from build123d import *

# Parameters (mm, degrees)
BOSS_EXTRUDE1_DEPTH = 9.8
LPATTERN1_COUNT     = 20
LPATTERN1_PITCH     = 11


with BuildPart() as part:
    # Sketch1 → Boss-Extrude1 (new body)
    with BuildSketch(Plane(origin=(0, 0, 0), x_dir=(0, 0, -1), z_dir=(1, 0, 0))):
        Polygon((0, 0), (4.8, 0), (11, 0), (11, 2.8), (4.8, 2.8), (4.8, 5.8), (0, 5.8), align=None)
    boss_extrude1 = extrude(amount=BOSS_EXTRUDE1_DEPTH)

    # LPattern1: Boss-Extrude1 ×20
    with Locations(*[(0, 0, -i * LPATTERN1_PITCH) for i in range(1, LPATTERN1_COUNT)]):
        add(boss_extrude1)


solid = part.part
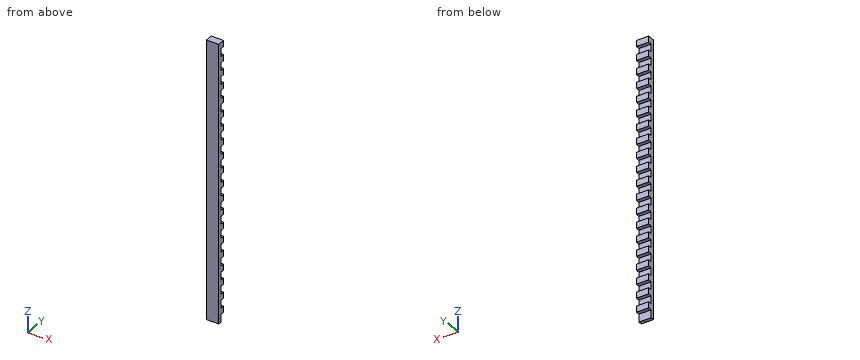
CAD build for the part. Positions are in the model's coordinates, mm. Round coordinates to 2 decimals unless told otherwise and drop trailing zeros. Answer as a JSON object with one key per item and string values.
(1) Band-saw the part on A-A, the plane y = 4.4. Count the separate pieces of the cut face and the enclosed holes in it, then the cut area to 3 significant figures.
Reported:
{"separate pieces": "20", "enclosed holes": "0", "area": "941 mm^2"}
(2) Probe probe 1 along Y at (x, z) = (6, -141.5). List the from-to ranges inside material, lowest first. Write a range as [from, to].
Reported:
{"probe 1": "y = [0, 2.8]"}
(3) Pin check, flat tips, straight feed: P1, Ø1, axis at x = 3, z = -104.5, coming from the +Y side; P2, Ø0.9, axis at x = 4.5, y = 4, coming from the -Z side. Stop position of each tip, or through.
Reported:
{"P1": "stops at y = 2.8", "P2": "stops at z = -213.8"}
